Read the model definition and answer for the solid it produces. Units are mm, in the model's axes. A direction names the side the tool comes from. Give positions to 0.01 mm unless a question says otherwise; leave off trailing zeros. Write each loop counter-clockwise with the first axis right and the second up, starting at its lowest first coordinate (ties: lowest second). Pieces come first, ordered by that corner, then holes. Notation, with made-up numbers: (-16.5, -35) - (41.5, -35) arc R32 ccw to (41.5, 2) - close; hole circle Ø2 at (80.25, 79.5). An arc over 180 degrees is marked (long way). Answer as CSV lines item,"result".
```python
from build123d import *

# Parameters (mm, degrees)
SZKIC1_W                                           = 596
SZKIC1_H                                           = 268
DODANIE_WYCI_GNI_CIE1_DEPTH                        = 22
POG_BIENIE_WALCOWE_POD_M10_WKR_T_Z_BEM_D           = 11
POG_BIENIE_WALCOWE_POD_M10_WKR_T_Z_BEM_CBORE_D     = 18
POG_BIENIE_WALCOWE_POD_M10_WKR_T_Z_BEM_CBORE_DEPTH = 10.6
OTW_R_GWINTOWANY_M41_D                             = 3.3
OTW_R_GWINTOWANY_M41_DEPTH                         = 11.5
OTW_R_GWINTOWANY_M41_TIP                           = 0.991420021
OTW_R_GWINTOWANY_M161_D                            = 14


with BuildPart() as part:
    # Szkic1 → Dodanie-wyciągnięcie1 (new body)
    with BuildSketch(Plane(origin=(0, 0, 0), x_dir=(1, 0, 0), z_dir=(0, 1, 0))):
        with Locations((298, 134)):
            Rectangle(SZKIC1_W, SZKIC1_H)
    extrude(amount=DODANIE_WYCI_GNI_CIE1_DEPTH)

    # Pogłębienie walcowe pod M10 Wkręt z łbem walcowym z gniazdem sześciokątnym1 (through all)
    with Locations(Plane(origin=(66, 22, -254), x_dir=(0, 0, 1), z_dir=(0, 1, 0))):
        with Locations((0, 0), (240, 0), (240, 464), (0, 464)):
            CounterBoreHole(POG_BIENIE_WALCOWE_POD_M10_WKR_T_Z_BEM_D / 2, POG_BIENIE_WALCOWE_POD_M10_WKR_T_Z_BEM_CBORE_D / 2, POG_BIENIE_WALCOWE_POD_M10_WKR_T_Z_BEM_CBORE_DEPTH)

    # Otwór gwintowany M41
    with Locations(Plane(origin=(43, 22, -14), x_dir=(0, 0, 1), z_dir=(0, 1, 0))):
        with Locations((0, 0), (-240, 0), (-240, 510), (0, 510)):
            Hole(OTW_R_GWINTOWANY_M41_D / 2, depth=OTW_R_GWINTOWANY_M41_DEPTH)
            with Locations((0, 0, -(OTW_R_GWINTOWANY_M41_DEPTH + OTW_R_GWINTOWANY_M41_TIP / 2))):  # 118° drill point
                Cone(0, OTW_R_GWINTOWANY_M41_D / 2, OTW_R_GWINTOWANY_M41_TIP, mode=Mode.SUBTRACT)

    # Otwór gwintowany M161 (through all)
    with Locations(Plane(origin=(298, 22, -134), x_dir=(0, 0, 1), z_dir=(0, 1, 0))):
        with Locations((0, 0)):
            Hole(OTW_R_GWINTOWANY_M161_D / 2)


solid = part.part
```
(1) For faces 1 (the flat face through (62, 11.4, -258)), 2 (the flat face through (294, 11, -268)), determine the directions among +Z, -Z, +X, -X, +Y, -Y from which every point of the face is accessible in a straight line to the end or side of a thin tool.
Worked out:
face 1,"+Y"
face 2,"-Z, +X, -X, +Y, -Y"
(2) A cutting plane is placed at B-B (x = 66). Write down the section's boundary in (y, z).
Worked out:
outline,"(0, -268) - (22, -268) - (22, -263) - (11.4, -263) - (11.4, -259.5) - (0, -259.5) - close; (0, -248.5) - (11.4, -248.5) - (11.4, -245) - (22, -245) - (22, -23) - (11.4, -23) - (11.4, -19.5) - (0, -19.5) - close; (0, -8.5) - (11.4, -8.5) - (11.4, -5) - (22, -5) - (22, 0) - (0, 0) - close"
(3) Each of these flat-tipped pins is pushed along its axis until it touches: P1, Ø5.5, axis at x = 64.5, z = -16.5, coming from the +Y side; P2, Ø2.5, axis at x = 553, z = -14, coming from the +Y side; P3, Ø11, axis at x = 298, z = -134, coming from the -Y side. Where does it stop, or does it pass through?
Worked out:
P1,"stops at y = 11.4"
P2,"stops at y = 10.26"
P3,"passes through"
(4) A cutting plane is placed at A-A (z = -134). Write down the section's boundary in (x, y).
Worked out:
outline,"(0, 0) - (291, 0) - (291, 22) - (0, 22) - close; (305, 0) - (596, 0) - (596, 22) - (305, 22) - close"
(5) Find the intervals of material crossed by L1, parallel to Z at x = 530, y = 4.75; L2, parallel to X at y = 18, z = -14; L3, parallel to X at y = 3, z = -254, in increasing order.
Worked out:
L1,"z = -268 to -259.5, -248.5 to -19.5, -8.5 to 0"
L2,"x = 0 to 41.35, 44.65 to 57, 75 to 521, 539 to 551.35, 554.65 to 596"
L3,"x = 0 to 60.5, 71.5 to 524.5, 535.5 to 596"
(6) The mould has two halves that part along Z. Classify faces 3 (the flat face through (294, 11, 0)), 4 (the flat face through (0, 11, -132)), 5 (the cylindrical face through (525.1, 5.6, -256.5)), 6 (the flat face through (534, 11.4, -10)): +Z half, -Z half, draft (parallel to the pull), parting line (faces both ways), or undercut.
Worked out:
face 3,"+Z half"
face 4,"draft"
face 5,"undercut"
face 6,"undercut"
